Autodesk Inventor part; units mm, degrees
ref_plane "작업 평면1" through (0, 0, -41) normal (0, 0, 1) x (1, 0, 0)
ref_plane "작업 평면2" through (0, 0, -41) normal (0, 0, 1) x (1, 0, 0)
ref_plane "YZ Plane" through (0, 0, 0) normal (1, 0, 0) x (0, 1, 0)
sketch "스케치1" plane through (0, 0, 0) normal (0, 1, 0) x (-1, 0, 0)
  arc A0 (0, -41) -> (0, 41) centre (0, 0) ccw
  line L0 (0, 41) -> (0, -41)
  dimension "d0" = 82
extrude "돌출1" add sketch "스케치1" along normal mid plane 54
shell "쉘1" thickness 2 removed faces 1 at (0, 9, -13.6667)
sketch "스케치3" plane through (0, 27, 0) normal (0, 1, 0) x (1, 0, 0)
  circle A0 centre (0, 0) radius 22.25
  line L0 (0, 41) -> (0, -41)
  line L1 (0, -22.25) -> (0, 22.25)
  dimension "d4" = 44.5
extrude "돌출2" add sketch "스케치3" against normal blind 2 contours A0 L0 picked at (7.4489, 4.8102)
mirror "미러1" about plane through (0, 0, 0) normal (0, 1, 0) of "돌출2"
sketch "스케치4" plane through (0, 27, 0) normal (0, 1, 0) x (1, 0, 0)
  circle A0 centre (0, 0) radius 20
  dimension "d7" = 40
extrude "돌출3" add sketch "스케치4" along normal blind 5
sketch "스케치5" plane through (0, 32, 0) normal (0, 1, 0) x (1, 0, 0)
  circle A0 centre (0, 0) radius 2.5
  dimension "d10" = 5
extrude "돌출4" add sketch "스케치5" along normal blind 7
sketch "스케치6" plane through (0, -27, 0) normal (0, -1, 0) x (1, 0, 0)
  circle A0 centre (0, 0) radius 5.75
  dimension "d13" = 11.5
extrude "돌출5" add sketch "스케치6" along normal blind 13
sketch "스케치7" plane through (0, -40, 0) normal (0, -1, 0) x (1, 0, 0)
  circle A0 centre (0, 0) radius 2.5
  dimension "d16" = 5
extrude "돌출6" add sketch "스케치7" along normal blind 6
chamfer "모따기1" distance 2 angle 45 1 edges at (-5.75, -40, 0)
ref_plane "작업 평면1" through (0, 0, -41) normal (0, 0, 1) x (1, 0, 0)
sketch "스케치8" plane through (0, 0, -41) normal (0, 0, 1) x (1, 0, 0)
  circle A0 centre (0, 0) radius 20.5
  dimension "d23" = 41
extrude "돌출7" cut sketch "스케치8" along normal up to surface
ref_plane "작업 평면2" through (0, 0, -41) normal (0, 0, 1) x (1, 0, 0)
sketch "스케치9" plane through (0, 0, -41) normal (0, 0, 1) x (1, 0, 0)
  circle A0 centre (0, 0) radius 20.5
  line L0 (0, 25) -> (0, 20.5)
  line L1 (0, 20.5) -> (0, -20.5)
  dimension "d27" = 41
extrude "돌출8" add sketch "스케치9" along normal blind 6 contours L1 A0 picked at (-6.7835, -0.8237)
sketch "스케치10" plane through (0, 0, -41) normal (0, 0, -1) x (-1, 0, 0)
  circle A0 centre (0, 0) radius 20.25
  dimension "d30" = 40.5
extrude "돌출9" cut sketch "스케치10" against normal blind 10
sketch "스케치11" plane through (0, 0, -41) normal (0, 0, -1) x (-1, 0, 0)
  arc A0 (0, -25) -> (0, 25) centre (0, 0) ccw
  line L0 (0, 25) -> (0, 20.25)
  line L1 (0, -20.25) -> (0, -25)
  arc A1 (0, -20.25) -> (0, 20.25) centre (0, 0) ccw
extrude "돌출10" add sketch "스케치11" against normal up to surface
properties part number "헤드(상)"
For this review, take the finished solid that the model builds, in its own axes (mm). A direction names the side the tool comes from. Coordinates: 2 decimals unless noted, no trailing zeros. Order: outer loops, then holes, each group sorted by start corner. A loop starts at its lowest first (then second) coordinate and runs counter-clockwise, first axis right, second up. Notation, with made-up numbers: (-2, 11) - (42, 11) arc R28 cw to (42, 29) - close; hole circle Ø11 at (-8, -10.5). An arc over 180 degrees is marked (long way). Use one line per item in the form item = value.
Q1. Consider section B-B (z = 0). Give the boundary of the cut face in (x, y), then the cut area to 4 significant figures.
Checked values:
outline = (-41, -27) - (-5.75, -27) - (-5.75, -38) - (-3.75, -40) - (-2.5, -40) - (-2.5, -46) - (2.5, -46) - (2.5, -40) - (3.75, -40) - (5.75, -38) - (5.75, -27) - (22.25, -27) - (22.25, -25) - (-39, -25) - (-39, 25) - (22.25, 25) - (22.25, 27) - (20, 27) - (20, 32) - (2.5, 32) - (2.5, 39) - (-2.5, 39) - (-2.5, 32) - (-20, 32) - (-20, 27) - (-41, 27) - close
area = 763.5 mm2
Q2. For P1, Ø12, axis at x = -33.5, y = -27, coming from the -Z side; P2, Ø12, axis at x = -13, y = 15, coming from the +Z side; P3, Ø6, axis at x = -27.5, y = 24.5, coming from the -Z side, all flat-tipped, find the tip position at first contact; note any pin that passes through.
Checked values:
P1 = -30.41
P2 = 40.4
P3 = -32.87
Q3. Consider section D-D (x = -23). Give the boundary of the cut face in (y, z), then the cut area to 3 significant figures.
Checked values:
outline = (-27, -33.94) - (-9.8, -33.94) - (-9.8, -41) - (9.8, -41) - (9.8, -33.94) - (27, -33.94) - (27, 33.94) - (-27, 33.94) - close; hole (-25, -31.5) - (25, -31.5) - (25, 31.5) - (-25, 31.5) - close
area = 654 mm2
Q4. Consider section C-C (y = 0). Give the boundary of the cut face in (x, z), then the cut area to 3 significant figures.
Checked values:
outline = (-25, -41) - (-20.25, -41) - (-20.25, -35) - (-20.5, -35) - (-20.5, -33.18) arc R39 cw to (0, 39) - (0, 41) arc R41 ccw to (-25, -32.5) - close
area = 241 mm2
Q5. Draft analysis for pull direction Y (two halves, no side actions). For faces 6 (the cylindrical face through (-20.5, -0.2, -34.3)), 7 (the cylindrical face through (-0.75, -32.42, -5.7)), 8 (the flat face through (0, -40, 3)), state which applies: +Y half, -Y half, draft (parallel to the pull), parting line (faces both ways), or undercut.
Checked values:
face_6 = undercut
face_7 = draft
face_8 = -Y half
Q6. For faces 1 (the cylindrical face through (-20.245, -0.445, -38.042)), 2 (the flat face through (0, 25.2, -33.8)), 3 (the cylindrical face through (-24.994, -0.55, -37.752)), 4 (the cylindrical face through (-7.87, 18.93, -36.58)), 5 (the cylindrical face through (-0.54, 35.45, -2.44)), list the 3-axis set-ups (+Z, -Z, +X, -X, +Y, -Y) from which the entire face can be reached by the end or side of a thin tool; tool diameter is ignored.
Checked values:
face_1 = -Z, +X
face_2 = -Z, +X, +Y, -Y
face_3 = -Z, -X
face_4 = none
face_5 = +Y
Q7. Consider section A-A (x = 8). Give the boundary of the cut face in (y, z).
Checked values:
outline = (-27, -20.76) - (-25, -20.76) - (-25, 20.76) - (-27, 20.76) - close; (25, -20.76) - (27, -20.76) - (27, -18.33) - (32, -18.33) - (32, 18.33) - (27, 18.33) - (27, 20.76) - (25, 20.76) - close
Q8. For probe 1 along Y at (x, z) = (-1, 1.5); probe 2 along Y at (x, z) = (-20, 5.5); probe 3 along Z at (x, y) = (-20.5, 12), list the stretches that pass through material, from the lowest coordinate up. Write a range as from..to.
Checked values:
probe_1 = -46..-25, 25..39
probe_2 = -27..-25, 25..27
probe_3 = -41..-33.18, 33.18..35.51
